Could you check a few things on this model? Use its own coordinates, in mm. A direction names the side the tool comes from. Coordinates: 2 decimals unless noted, no trailing zeros. Order: outer loops, then holes, each group sorted by start corner. A loop starts at its lowest first (then second) coordinate and runs counter-clockwise, first axis right, second up. Notation, with made-up numbers: (45.25, -15) -> (58.25, -15) arc R23 ccw to (58.25, 23) -> close; hole circle Ø2 at (78.5, 8). An arc over 180 degrees is marked (long way). Use a Markdown table: item, result. Add a question column.
1) If we section it at C-C (x = -3.5): Write out the boundary of the cut face in (y, z), plus the area to 3 significant figures.
2) If I drill on L1, parallel to Y at x = -14.55, z = 10; L2, parallel to Y at x = -9.5, z = 3; L3, parallel to X at y = 19, z = 6, over which ranges is the centre line in solid material (lowest first)? Write a range as [from, to].
3) If we section it at A-A (z = 10): Write out the boundary of the cut face in (x, y).
4) If we section it at B-B (y = 25.5): Write out the boundary of the cut face in (x, z), plus the area to 3 significant figures.
5) Which directions (+Z, -Z, +X, -X, +Y, -Y) give clear straight access to the entire face, cutting with the end or side of a thin tool? Please do faces 5 (the cylindrical face through (0.2, 22.7, 7.05)), 6 (the flat face through (14, 20, 10)), 7 (the flat face through (-14, 20, 10)), 8 (the flat face through (0, -27, 10)).
6) Thinking about a two-plate mould opening in Z: for faces 1 (the flat face through (0, 27, 10)), 2 (the flat face through (-15, 2, 0)), 3 (the cylindrical face through (15.52, 21.01, 11.11)), 4 (the flat face through (-15, 2, 20)), which applies, +Z half, -Z half, draft (parallel to the pull), parting line (faces both ways), or undercut?
7) Will these pins go through, and if not, where does the flat tip stop? pin 1 Ø2.5 at (y, z) = (20, 10) entering from +X; pin 2 Ø1.5 at (y, z) = (20, 10.5) entering from -X; pin 3 Ø5 at (x, y) = (8, 21.5) entering from -Z.
8) If we section it at D-D (z = 18.75): Write out the boundary of the cut face in (x, y), plus the area to 3 significant figures.
```python
from build123d import *

# Parameters (mm, degrees)
SKETCH1_W               = 34
SKETCH1_H               = 60
SKETCH1_W_2             = 28
SKETCH1_H_2             = 54
BOSS_EXTRUDE1_DEPTH     = 20
SKETCH2_R               = 1.5
CUT_EXTRUDE1_DEPTH      = 1
CUT_EXTRUDE1_DEPTH_BACK = 35
SKETCH4_R               = 4
BOSS_EXTRUDE2_DEPTH     = 28


with BuildPart() as part:
    # Sketch1 → Boss-Extrude1 (new body)
    with BuildSketch(Plane.XY):
        Rectangle(SKETCH1_W, SKETCH1_H)
        Rectangle(SKETCH1_W_2, SKETCH1_H_2, mode=Mode.SUBTRACT)
    extrude(amount=BOSS_EXTRUDE1_DEPTH)

    # Sketch2 → Cut-Extrude1 (cut, two sides)
    with BuildSketch(Plane(origin=(17, 0, 0), x_dir=(0, 0, -1), z_dir=(1, 0, 0))) as cut_extrude1_sk:
        with Locations((-10, -22.5)):
            Circle(SKETCH2_R)
        with Locations((-10, 20)):
            Circle(SKETCH2_R)
    extrude(amount=CUT_EXTRUDE1_DEPTH, mode=Mode.SUBTRACT)
    extrude(cut_extrude1_sk.sketch, amount=-CUT_EXTRUDE1_DEPTH_BACK, mode=Mode.SUBTRACT)

    # Sketch4 → Boss-Extrude2 (add)
    with BuildSketch(Plane.ZY.offset(-14)):
        with Locations((10, 20)):
            Circle(SKETCH4_R)
    extrude(amount=BOSS_EXTRUDE2_DEPTH)


solid = part.part
```
Answer sheet:
| question | item | result |
|---|---|---|
| 1 | outline | (-30, 0) -> (-27, 0) -> (-27, 20) -> (-30, 20) -> close; circle Ø8 at (20, 10); (27, 0) -> (30, 0) -> (30, 20) -> (27, 20) -> close |
| 1 | area | 170 mm2 |
| 2 | L1 | [-30, -24], [-21, 18.5], [21.5, 30] |
| 2 | L2 | [-30, -27], [27, 30] |
| 2 | L3 | [-17, -14], [14, 17] |
| 3 | outline | (-17, -30) -> (17, -30) -> (17, -24) -> (14, -24) -> (14, -27) -> (-14, -27) -> (-14, -24) -> (-17, -24) -> close; (-17, -21) -> (-14, -21) -> (-14, 16) -> (14, 16) -> (14, -21) -> (17, -21) -> (17, 18.5) -> (14, 18.5) -> (14, 21.5) -> (17, 21.5) -> (17, 30) -> (-17, 30) -> (-17, 21.5) -> (-14, 21.5) -> (-14, 18.5) -> (-17, 18.5) -> close; hole (-14, 24) -> (14, 24) -> (14, 27) -> (-14, 27) -> close |
| 4 | outline | (-17, 0) -> (-14, 0) -> (-14, 20) -> (-17, 20) -> close; (14, 0) -> (17, 0) -> (17, 20) -> (14, 20) -> close |
| 4 | area | 120 mm2 |
| 5 | face 5 | none |
| 5 | face 6 | +X |
| 5 | face 7 | -X |
| 5 | face 8 | +Z, -Z |
| 6 | face 1 | draft |
| 6 | face 2 | -Z half |
| 6 | face 3 | undercut |
| 6 | face 4 | +Z half |
| 7 | pin 1 | x = 14 |
| 7 | pin 2 | x = -14 |
| 7 | pin 3 | z = 6 |
| 8 | outline | (-17, -30) -> (17, -30) -> (17, 30) -> (-17, 30) -> close; hole (-14, -27) -> (14, -27) -> (14, 27) -> (-14, 27) -> close |
| 8 | area | 528 mm2 |
